```python
from build123d import *

# Parameters (mm, degrees)
EXTRUDE_1_DEPTH     = 20
SKETCH_2_R          = 2.5
CUT_EXTRUDE_1_DEPTH = 4
SKETCH_3_R          = 3
CUT_EXTRUDE_2_DEPTH = 4


with BuildPart() as part:
    # Эскиз1 → Бобышка-Вытянуть1 (new body)
    with BuildSketch(Plane(origin=(0, 0, 0), x_dir=(1, 0, 0), z_dir=(0, 1, 0))):
        Polygon((50, 0), (170, 43.676428112), (170, 47.933139202), (49.294692077, 4), (4, 4), (4, 20.7), (0, 20.7), (0, 4), (0, 0), align=None)
    extrude(amount=EXTRUDE_1_DEPTH)

    # Эскиз2 → Вырез-Вытянуть1 (cut)
    with BuildSketch(Plane.ZY):
        with Locations((-10, 5)):
            Circle(SKETCH_2_R)
        with Locations((-10, 15)):
            Circle(SKETCH_2_R)
    extrude(amount=-CUT_EXTRUDE_1_DEPTH, mode=Mode.SUBTRACT)

    # Эскиз3 → Вырез-Вытянуть2 (cut)
    with BuildSketch(Plane.XY):
        with Locations((21, 10.690090477)):
            Circle(SKETCH_3_R)
    extrude(amount=-CUT_EXTRUDE_2_DEPTH, mode=Mode.SUBTRACT)


solid = part.part
```
Part model, mm, in its own coordinate system. A direction names the side the tool comes from. Round coordinates to 2 decimals unless told otherwise and drop trailing zeros. Loops run counter-clockwise (first coordinate to the right, second up) from the corner with the lowest first, then second, coordinate; pieces in that order, holes last.
Item 1: Cut at C-C, the plane z = -40. Give the cut face in (x, y).
Item 2: Drill centre lines: line 1 (Y direction, x = 1.25, z = -10); line 2 (Z direction, x = 9, y = 5); line 3 (Z direction, x = 82.5, y = 13.5). Where is each one in solid material? Low to high.
Item 3: Mould opens along X. For faces 6 (the face through (2, 13.5, -12)), 7 (the face through (4, 10, -12)), 8 (the face through (110.492, 9.86, -26.274)), 9 (the face through (109.16, 9.86, -21.532)) say: +X half, -X half, draft (parallel to the pull), parting line (faces both ways), or undercut.
Item 4: Cut at B-B, the plane x = 21. Give the cut face in (y, z), then the cut area to 3 significant figures.
Item 5: Cut at A-A, the plane y = 5. Give the cut face in (x, z).
Item 6: Cut at D-D, the plane x = 66. Give the cut face in (y, z).
Item 7: Drop flat-ended pins along their axis: P1, Ø3.5, axis at x = 21, y = 10.69, coming from the +Z side; P2, Ø10, axis at x = 67.5, y = 10.5, coming from the -Z side; P3, Ø1.5, axis at x = 141.5, y = 17.5, coming from the -Z side; P4, Ø1, axis at x = 132, y = 6.5, coming from the -Z side. Give the stop position or say it passes through.
Item 8: 3-axis set-ups, long thin cutter, end or side, ignore diameter. For faces 1 (the face through (27, 10, -4)), 2 (the face through (0, 10, -10)), 3 (the face through (1.97, 6.69, -11.84)), 4 (the face through (2, 10, -20.7)), 5 (the face through (25, 10, 0)): which of +Z, -Z, +X, -X, +Y, -Y reach the whole face in a straight line?
A:
1. outline: (148.2, 0) - (159.9, 0) - (159.9, 20) - (148.2, 20) - close
2. line 1: y = 0 to 2.5, 7.5 to 12.5, 17.5 to 20
2. line 2: z = -4 to 0
2. line 3: z = -16.09 to -11.83
3. face 6: draft
3. face 7: undercut
3. face 8: undercut
3. face 9: +X half
4. outline: (0, -4) - (7.69, -4) - (7.69, 0) - (0, 0) - close; (13.69, -4) - (20, -4) - (20, 0) - (13.69, 0) - close
4. area: 56.0 mm2
5. outline: (0, -20.7) - (4, -20.7) - (4, -12.5) - (0, -12.5) - close; (0, -7.5) - (4, -7.5) - (4, -4) - (49.29, -4) - (170, -47.93) - (170, -43.68) - (50, 0) - (0, 0) - close
6. outline: (0, -10.08) - (20, -10.08) - (20, -5.82) - (0, -5.82) - close
7. P1: passes through
7. P2: stops at z = -12.45
7. P3: stops at z = -37.83
7. P4: stops at z = -34.28
8. face 1: -Z, +Y, -Y
8. face 2: +Z, -Z, -X, +Y, -Y
8. face 3: -X
8. face 4: -Z, -X, +Y, -Y
8. face 5: +Z, +X, -X, +Y, -Y
